Part model, mm, in its own coordinate system. A direction names the side the tool comes from. Give positions to 0.01 mm unless a question says otherwise; leave off trailing zeros. Write each loop counter-clockwise with the first axis right and the second up, starting at its lowest first coordinate (ties: lowest second). Pieces come first, ordered by that corner, then holes.
from build123d import *

# Parameters (mm, degrees)
F1_DEPTH = 12
F2_R     = 6
F3_DEPTH = 6
F4_R     = 2.5
F5_DEPTH = 31.5


with BuildPart() as f1:
    # F0 (on Top) → F1 (new body)
    with BuildSketch(Plane.XY):
        with BuildLine():
            Line((-7, -13), (7, -13))
            ThreePointArc((7, -13), (11.242641, -11.242641), (13, -7))
            Line((13, -7), (13, 7))
            ThreePointArc((13, 7), (11.242641, 11.242641), (7, 13))
            Line((7, 13), (-7, 13))
            ThreePointArc((-7, 13), (-11.242641, 11.242641), (-13, 7))
            Line((-13, 7), (-13, -7))
            ThreePointArc((-13, -7), (-11.242641, -11.242641), (-7, -13))
        make_face()
    extrude(amount=F1_DEPTH)

    # F2 (on face) → F3 (cut)
    with BuildSketch(Plane.XY.offset(12)):
        Circle(F2_R)
    extrude(amount=-F3_DEPTH, mode=Mode.SUBTRACT)

    # F4 (on face) → F5 (cut)
    with BuildSketch(Plane.XY.offset(6)):
        Circle(F4_R)
    extrude(amount=-F5_DEPTH, mode=Mode.SUBTRACT)


solid = f1.part
1) Saw through at A-A (x = 0). Write the cut outline in (y, z), and give its area (3 significant figures).
Check result:
outline: (-13, 0) - (-2.5, 0) - (-2.5, 6) - (-6, 6) - (-6, 12) - (-13, 12) - close; (2.5, 0) - (13, 0) - (13, 12) - (6, 12) - (6, 6) - (2.5, 6) - close
area: 210 mm2
2) Mould opens along X. For faces 1 (the flat face through (13, 0, 6)), 2 (the flat face through (3, 0, 6)), 3 (the flat face through (6, 3, 12)) say: +X half, -X half, draft (parallel to the pull), parting line (faces both ways), or undercut.
Check result:
face 1: +X half
face 2: undercut
face 3: draft
3) Flat gauge pins, fed straight in: P1, Ø3, axis at x = -9.5, z = 6.5, coming from the -Y side; P2, Ø2, axis at x = 3.5, y = 3, coming from the +Z side; P3, Ø6, axis at x = -3, y = 1.5, coming from the +Z side. Where does each tip first touch, or does it go through?
Check result:
P1: stops at y = -12.92
P2: stops at z = 6
P3: stops at z = 12
4) 3-axis set-ups, long thin cutter, end or side, ignore diameter. For faces 4 (the cylindrical face through (-6, 0, 9)), 5 (the flat face through (-13, 0, 6)): which of +Z, -Z, +X, -X, +Y, -Y reach the whole face in a straight line?
Check result:
face 4: +Z
face 5: +Z, -Z, -X, +Y, -Y
5) Saw through at C-C (z = 7). Write the cut outline in (x, y), and give its area (3 significant figures).
Check result:
outline: (-13, -7) arc R6 ccw to (-7, -13) - (7, -13) arc R6 ccw to (13, -7) - (13, 7) arc R6 ccw to (7, 13) - (-7, 13) arc R6 ccw to (-13, 7) - close; hole circle Ø12 at (0, 0)
area: 532 mm2
6) Saw through at D-D (x = -4). Write the cut outline in (y, z), and give its area (3 significant figures).
Check result:
outline: (-13, 0) - (13, 0) - (13, 12) - (4.47, 12) - (4.47, 6) - (-4.47, 6) - (-4.47, 12) - (-13, 12) - close
area: 258 mm2
7) Drill centre lines: L1, parallel to Y at x = 0, z = 1.4; L2, parallel to Y at x = 0, z = 7.35; L3, parallel to X at y = -4.75, z = 7.5. Where is each one in solid material? Low to high.
Check result:
L1: y = -13 to -2.5, 2.5 to 13
L2: y = -13 to -6, 6 to 13
L3: x = -13 to -3.67, 3.67 to 13
